Autodesk Fusion 360 part; units mm, degrees
sketch "Skizze1" plane through (0, 0, 0) normal (0, 1, 0) x (1, 0, 0)
  line L0 (0, 0) -> (40, 0)
  line L1 (40, 0) -> (40, -10)
  line L2 (40, -10) -> (0, -10)
  line L3 (0, 0) -> (0, -10)
extrude "Extrusion1" add sketch "Skizze1" along normal blind 15
sketch "Skizze2" plane through (0, 15, 0) normal (0, 1, 0) x (-1, 0, 0)
  line L0 (-40, 0) -> (0, 0)
  line L1 (0, 0) -> (0, 10)
  line L2 (0, 10) -> (-40, 10)
  line L3 (-40, 10) -> (-40, 0)
  line L4 (0, 0) -> (-10, 0)
  circle A0 centre (-10, 5) radius 1.5
  circle A1 centre (-30, 5) radius 1.5
  dimension "d3" = 3
  dimension "d4" = 3
extrude "Extrusion2" cut sketch "Skizze2" against normal blind 40 contours A0 | A1
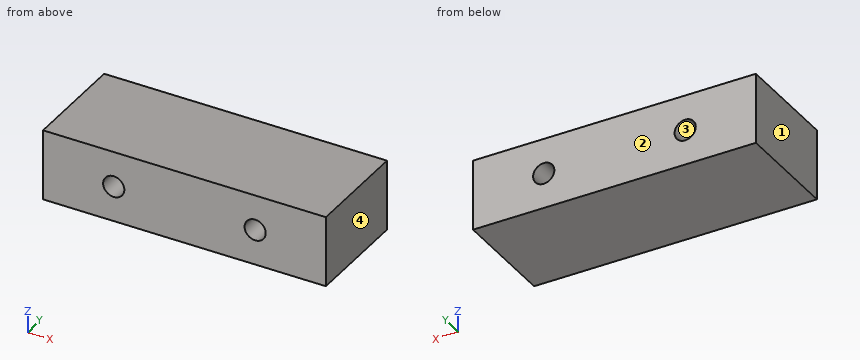
Part model, mm, in its own coordinate system. Face numbers are marked on the shaded views. Round coordinates to 2 decimals unless told otherwise and drop trailing zeros. Write each loop counter-clockwise with the first axis right and the second up, starting at its lowest first coordinate (ties: lowest second). Pieces come first, ordered by that corner, then holes. Notation, with made-up numbers: M 75.25,47 L 88.25,47 A30 ccw 88.25,77 Z; hole C 33,-23.5 d3. An arc over 180 degrees is marked long. One line per question, with ' | ' between items.
(1) Saw through at C-C on y = 10.5. Write the cut outline in (x, z).
Answer key:
outline: M 0,0 L 40,0 L 40,10 L 0,10 Z; hole C 10,5 d3; hole C 30,5 d3
(2) Saw through at A-A on x = 30. Write the cut outline in (y, z), then the cut area to 3 significant figures.
Answer key:
outline: M 0,0 L 15,0 L 15,3.5 L 0,3.5 Z; M 0,6.5 L 15,6.5 L 15,10 L 0,10 Z | area: 105 mm^2
(3) Saw through at B-B on z = 5. Write the cut outline in (x, y).
Answer key:
outline: M 0,0 L 8.5,0 L 8.5,15 L 0,15 Z; M 11.5,0 L 28.5,0 L 28.5,15 L 11.5,15 Z; M 31.5,0 L 40,0 L 40,15 L 31.5,15 Z
(4) Pin check, flat tip, straight feed: pin 1 (2.5 mm diameter, centred on x = 30, z = 5, fed in from +Y). Stop position of the tip, or through.
Answer key:
pin 1: passes through
(5) Probe line 1 along Z through (x, y) = (30, 8.5). List the from-to ranges inside material, lowest first.
Answer key:
line 1: z = 0 to 3.5, 6.5 to 10
(6) Two-plate mould, pull along X, no slides. Class the marked faces 1, 2, 3 and 4: released by +X, released by -X, zero draft, split by the parting line, or undercut.
Answer key:
face 1: released by -X | face 2: zero draft | face 3: undercut | face 4: released by +X
